Check sheet for the modelled part. Datum: model origin and axes. Units: mm. Round coordinates to 2 decimals unless told otherwise and drop trailing zeros. Write each loop counter-clockwise with the first axis right and the second up, starting at its lowest first coordinate (ties: lowest second). Pieces come first, ordered by that corner, then holes.
Item 1: Depth check by flat-ended pin: pin 1 (6.5 mm diameter, centred on x = 12.62, z = -15.36, fed in from +Y); pin 2 (1.8 mm diameter, centred on x = 13.62, z = 10.86, fed in from -Y). Enter the tip coordinate at first touch or a pass-through.
Item 2: Section check A-A, the plane x = -45. Record the cut outline in (y, z).
Item 3: Section check B-B, the plane y = 2.15. State how many separate pieces and enclosed holes the cut face has, plus the area to 3 significant figures.
Item 4: Material ranges on line 1 along Z through (x, y) = (-45, 0.85); line 2 along X through (y, z) = (0.25, 15); line 3 along Z through (x, y) = (0, 2.45), recorded low to high.
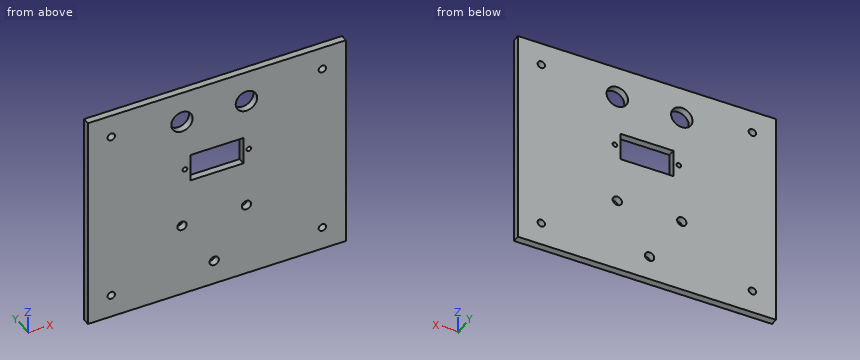
from build123d import *

# Parameters (mm, degrees)
SKETCH1_W           = 110
SKETCH1_H           = 95
SKETCH1_R           = 2
BOSS_EXTRUDE1_DEPTH = 3
SKETCH2_R           = 1.6
CUT_EXTRUDE1_DEPTH  = 3
SKETCH4_R           = 4.575
CUT_EXTRUDE3_DEPTH  = 3
SKETCH5_R           = 1
SKETCH5_W           = 22.5
SKETCH5_H           = 12
CUT_EXTRUDE4_DEPTH  = 10


with BuildPart() as part:
    # Sketch1 → Boss-Extrude1 (new body)
    with BuildSketch(Plane(origin=(0, 0, 0), x_dir=(1, 0, 0), z_dir=(0, 1, 0))):
        Rectangle(SKETCH1_W, SKETCH1_H)
        with Locations((-1.134990048, 36.85560657)):
            Circle(SKETCH1_R, mode=Mode.SUBTRACT)
        with Locations((-14.884990048, 15.35560657)):
            Circle(SKETCH1_R, mode=Mode.SUBTRACT)
        with Locations((12.615009952, 15.35560657)):
            Circle(SKETCH1_R, mode=Mode.SUBTRACT)
    extrude(amount=BOSS_EXTRUDE1_DEPTH)

    # Sketch2 → Cut-Extrude1 (cut)
    with BuildSketch(Plane(origin=(0, 3, 0), x_dir=(1, 0, 0), z_dir=(0, 1, 0))):
        with Locations((-45, 37.5)):
            Circle(SKETCH2_R)
        with Locations((45, 37.5)):
            Circle(SKETCH2_R)
        with Locations((-45, -37.5)):
            Circle(SKETCH2_R)
        with Locations((45, -37.5)):
            Circle(SKETCH2_R)
    extrude(amount=-CUT_EXTRUDE1_DEPTH, mode=Mode.SUBTRACT)

    # Sketch4 → Cut-Extrude3 (cut)
    with BuildSketch(Plane(origin=(0, 3, 0), x_dir=(1, 0, 0), z_dir=(0, 1, 0))):
        with Locations((-14.884990048, -33.869690938)):
            Circle(SKETCH4_R)
        with Locations((12.615009952, -33.869690938)):
            Circle(SKETCH4_R)
    extrude(amount=-CUT_EXTRUDE3_DEPTH, mode=Mode.SUBTRACT)

    # Sketch5 → Cut-Extrude4 (cut)
    with BuildSketch(Plane(origin=(0, 3, 0), x_dir=(1, 0, 0), z_dir=(0, 1, 0))):
        with Locations((-13.625, -10.858715864)):
            Circle(SKETCH5_R)
        with Locations((13.625, -10.858715864)):
            Circle(SKETCH5_R)
        with Locations((0, -10.858715864)):
            Rectangle(SKETCH5_W, SKETCH5_H)
    extrude(amount=-CUT_EXTRUDE4_DEPTH, mode=Mode.SUBTRACT)


solid = part.part
Values found:
1. pin 1: stops at y = 3
1. pin 2: passes through
2. outline: (0, -47.5) - (3, -47.5) - (3, -39.1) - (0, -39.1) - close; (0, -35.9) - (3, -35.9) - (3, 35.9) - (0, 35.9) - close; (0, 39.1) - (3, 39.1) - (3, 47.5) - (0, 47.5) - close
3. separate pieces: 1
3. enclosed holes: 12
3. area: 9,970 mm2
4. line 1: z = -47.5 to -39.1, -35.9 to 35.9, 39.1 to 47.5
4. line 2: x = -55 to -11.25, 11.25 to 55
4. line 3: z = -47.5 to -38.5, -35.21 to 4.86, 16.86 to 47.5
